```python
from build123d import *

# Parameters (mm, degrees)
EXTRUDE_2_DEPTH     = 15
FILLET_2_R          = 3
SKETCH_6_R          = 2.1
CUT_EXTRUDE_5_DEPTH = 13.55
SKETCH_7_R          = 2.1
CUT_EXTRUDE_6_DEPTH = 13.55
CUT_EXTRUDE_7_DEPTH = 2.55
CUT_EXTRUDE_8_DEPTH = 2.55


with BuildPart() as part:
    # Эскиз1 → Бобышка-Вытянуть2 (new body)
    with BuildSketch(Plane.XY):
        with BuildLine():
            Line((-34.742798859, 11.871098047), (-33.477492737, 10.322227357))
            Line((-33.477492737, 10.322227357), (-31.579533553, 7.998921321))
            Line((-31.579533553, 7.998921321), (-21.106042067, 13.856051683))
            Line((-21.106042067, 13.856051683), (-22.484178739, 17.02551412))
            ThreePointArc((-22.484178739, 17.02551412), (-3.742798859, 20.923766125), (14.99858102, 17.02551412))
            Line((14.99858102, 17.02551412), (13.620444348, 13.856051683))
            Line((13.620444348, 13.856051683), (24.062716277, 7.960705226))
            Line((24.062716277, 7.960705226), (25.991895018, 10.322227357))
            Line((25.991895018, 10.322227357), (27.257201141, 11.871098047))
            ThreePointArc((27.257201141, 11.871098047), (-3.742798859, 22.923766125), (-34.742798859, 11.871098047))
        make_face()
    extrude(amount=EXTRUDE_2_DEPTH)

    # Скругление2
    fillet_2_edges = [part.edges().sort_by_distance(p)[0] for p in [
        (14.99858102, 17.02551412, 7.5),
        (-22.484178739, 17.02551412, 7.5),
    ]]
    fillet(fillet_2_edges, radius=FILLET_2_R)

    # Эскиз6 → Вырез-Вытянуть5 (cut)
    with BuildSketch(Plane(origin=(9.223958982, 16.338155636, 0), x_dir=(0.8708059042632018, -0.4916269694599224, 0), z_dir=(-0.49162696945992235, -0.8708059042632017, 0))):
        with Locations((11.048754659, 7.5)):
            Circle(SKETCH_6_R)
    extrude(amount=-CUT_EXTRUDE_5_DEPTH, mode=Mode.SUBTRACT)

    # Эскиз7 → Вырез-Вытянуть6 (cut)
    with BuildSketch(Plane(origin=(-10.930954108, 19.546304709, 0), x_dir=(0.8727909572035157, 0.48809419687573696, 0), z_dir=(0.488094196875737, -0.8727909572035158, 0))):
        with Locations((-17.65810424, 7.409111806)):
            Circle(SKETCH_7_R)
    extrude(amount=-CUT_EXTRUDE_6_DEPTH, mode=Mode.SUBTRACT)

    # Эскиз8 → Вырез-Вытянуть7 (cut)
    with BuildSketch(Plane(origin=(-10.930954108, 19.546304709, 0), x_dir=(0.8727909572035158, 0.488094196875737, 0), z_dir=(0.488094196875737, -0.8727909572035158, 0))):
        Polygon((-19.707697696, 3.859111806), (-15.608510784, 3.859111806), (-13.558917329, 7.409111806), (-15.608510784, 10.959111806), (-19.707697696, 10.959111806), (-21.757291151, 7.409111806), align=None)
    extrude(amount=-CUT_EXTRUDE_7_DEPTH, mode=Mode.SUBTRACT)

    # Эскиз9 → Вырез-Вытянуть8 (cut)
    with BuildSketch(Plane(origin=(9.223958982, 16.338155636, 0), x_dir=(0.8708059042632018, -0.49162696945992246, 0), z_dir=(-0.4916269694599224, -0.8708059042632017, 0))):
        Polygon((8.999161204, 3.95), (13.098348115, 3.95), (15.147941571, 7.5), (13.098348115, 11.05), (8.999161204, 11.05), (6.949567748, 7.5), align=None)
    extrude(amount=-CUT_EXTRUDE_8_DEPTH, mode=Mode.SUBTRACT)


solid = part.part
```
Verification items for the finished model (mm, model axes). A direction names the side the tool comes from. Coordinates: 2 decimals unless noted, no trailing zeros. Order: outer loops, then holes, each group sorted by start corner. A loop starts at its lowest first (then second) coordinate and runs counter-clockwise, first axis right, second up. Notation, with made-up numbers: (-29.75, -5.5) - (28.25, -5.5) arc R24 ccw to (28.25, 28.5) - close; hole circle Ø7 at (41.5, 89). An arc over 180 degrees is marked (long way). Return JSON: item names as keys, results as strings.
(1) Section check B-B, the plane x = 0. Record the cut outline in (y, z), and give its area (3 significant figures).
Filled sheet:
{"outline": "(20.77, 0) - (22.78, 0) - (22.78, 15) - (20.77, 15) - close", "area": "30.1 mm^2"}
(2) Mould release check, pull along Z, two halves, no side actions. Record for faces 1 (the flat face through (-24.286, 13.518, 5.609)), 2 (the cylindrical face through (-3.968, 20.923, 7.395)): pulls with the +Z half, pulls with the -Z half, needs draft (parallel to the pull), parting line crosses it, or undercut.
Filled sheet:
{"face 1": "undercut", "face 2": "needs draft"}
(3) Go/stop test with flat-tipped pins: pin 1 (5 mm diameter, centred on y = 13, z = 2.5, fed in from -X); pin 2 (1.3 mm diameter, centred on x = 19.5, y = 11, fed in from -Z); pin 3 (1 mm diameter, centred on y = 17.5, z = 8.5, fed in from +X); pin 4 (8 mm diameter, centred on x = 0.5, z = 2, fed in from +Y). Record where each tip stops, or that it passes through.
Filled sheet:
{"pin 1": "stops at x = -34.74", "pin 2": "stops at z = 0", "pin 3": "stops at x = 19.61", "pin 4": "stops at y = 22.92"}
(4) Section check A-A, the plane z = 8.5. Record the cut outline in (x, y), and give its area (3 significant figures).
Filled sheet:
{"outline": "(-34.74, 11.87) - (-31.58, 8) - (-29.37, 9.23) - (-30.62, 11.46) - (-29.15, 12.28) - (-30.62, 14.9) arc R49 ccw to start; (-27.55, 16.75) - (-26.02, 14.03) - (-24.56, 14.85) - (-23.31, 12.62) - (-21.11, 13.86) - (-21.25, 14.18) arc R3 cw to (-19.5, 18.2) arc R47 cw to (12.02, 18.2) arc R3 cw to (13.76, 14.18) - (13.62, 13.86) - (15.78, 12.64) - (17.03, 14.86) - (18.49, 14.03) - (20.03, 16.77) arc R49 ccw to start; (21.71, 12.22) - (23.17, 11.4) - (21.91, 9.17) - (24.06, 7.96) - (27.26, 11.87) arc R49 ccw to (23.2, 14.85) - close", "area": "165 mm^2"}
(5) Thickness scan on line 1 along X through (y, z) = (14.25, 5.75); line 2 along X through (y, z) = (13.5, 6); line 3 along Y through (x, z) = (-3, 14.5). Record the ranges inside material, lowest first.
Filled sheet:
{"line 1": "x = -31.58 to -29.68, -26.73 to -25.63, -24.6 to -21.28, 13.79 to 17.19, 18.11 to 19.4, 22.07 to 24.09", "line 2": "x = -32.63 to -29.57, -24.02 to -21.74, 14.25 to 16.6, 22 to 25.15", "line 3": "y = 20.92 to 22.92"}
(6) Access from +Z, -Z, +X, -X, +Y, -Y to the whole of each face (thin tool, end or side, straight path). Record for faces 3 (the flat face through (-24.26, 13.53, 9.16)), 4 (the flat face through (-24.089, 12.188, 10.728)), 5 (the flat face through (-29.652, 10.517, 5.659)).
Filled sheet:
{"face 3": "-Y", "face 4": "+Z, -Z, -Y", "face 5": "none"}
(7) Section check C-C, the plane y = 21.5. Record the cut outline in (x, z).
Filled sheet:
{"outline": "(-15.47, 0) - (7.98, 0) - (7.98, 15) - (-15.47, 15) - close"}
